Source: three-view drawing plus pictorial views. Frame: mm from the lowest corner of the part. A direction names the side the tool comes from. Give positions to 0.01 mm unless a question says otherwise; leave off trailing zeros. Loops run counter-clockwise (first coordinate to the right, second up) from the corner with the lowest first, then second, coordinate; pieces in that order, holes last.
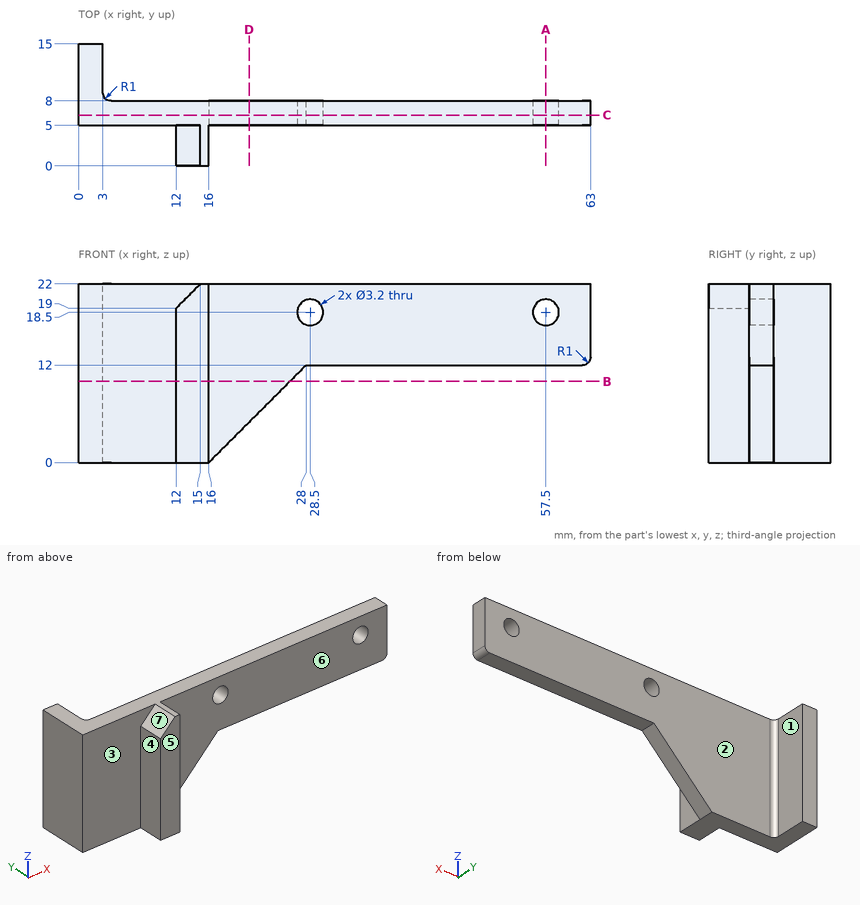
Q1. Material intervals for probe 1 along Z at (x, y) = (28.5, 5.6); probe 2 along Y at (x, z) = (8.5, 19.5); probe 3 along Z at (x, y) = (52, 7.5), sorted ascending.
Q2. Section query B-B, the plane z = 10. Return loops of the section in (x, y).
Q3. Reachability of the marked faces 4, 5, 6 and 7 from +Z, -Z, +X, -X, +Y, -Y: full face, straight path, thin tool, end or side. Return the list, or none.
Q4. Section query D-D, the plane x = 21. Return loops of the section in (y, z).
Q5. Pin query (flat end, axial travel): pin 1 Ø4.5 at (x, z) = (9, 9) entering from -Y; pin 2 Ø2 at (x, z) = (22.5, 16) entering from +Y; pin 3 Ø1.8 at (y, z) = (11.5, 16.5) entering from +X. Return the tip coordinate at first contact, or that it passes through.
Q6. Section query A-A, the plane x = 57.5. Return loops of the section in (y, z).
Q7. Section query C-C, the plane y = 6.25. Return loops of the section in (x, z), and give its area (3 significant figures).
Q8. Mould query, pull axis Y, two halves, no side actions, for the marked faces 1, 2 and 3. Classes: +Y half, -Y half, draft (parallel to the pull), parting line (faces both ways), or undercut.
Resolved:
1. probe 1: z = 12 to 16.9, 20.1 to 22
1. probe 2: y = 5 to 8
1. probe 3: z = 12 to 22
2. outline: (0, 5) - (12, 5) - (12, 0) - (16, 0) - (16, 5) - (26, 5) - (26, 8) - (4, 8) arc R1 cw to (3, 9) - (3, 15) - (0, 15) - close
3. face 4: +Z, -Z, -X, -Y
3. face 5: +Z, -Z, +X, -X, -Y
3. face 6: +Z, -Z, +X, -Y
3. face 7: +Z, -X, -Y
4. outline: (5, 5) - (8, 5) - (8, 22) - (5, 22) - close
5. pin 1: stops at y = 5
5. pin 2: stops at y = 8
5. pin 3: stops at x = 3
6. outline: (5, 12) - (8, 12) - (8, 16.9) - (5, 16.9) - close; (5, 20.1) - (8, 20.1) - (8, 22) - (5, 22) - close
7. outline: (0, 0) - (16, 0) - (28, 12) - (62, 12) arc R1 ccw to (63, 13) - (63, 22) - (0, 22) - close; hole circle Ø3.2 at (28.5, 18.5); hole circle Ø3.2 at (57.5, 18.5)
7. area: 878 mm2
8. face 1: draft
8. face 2: +Y half
8. face 3: -Y half
